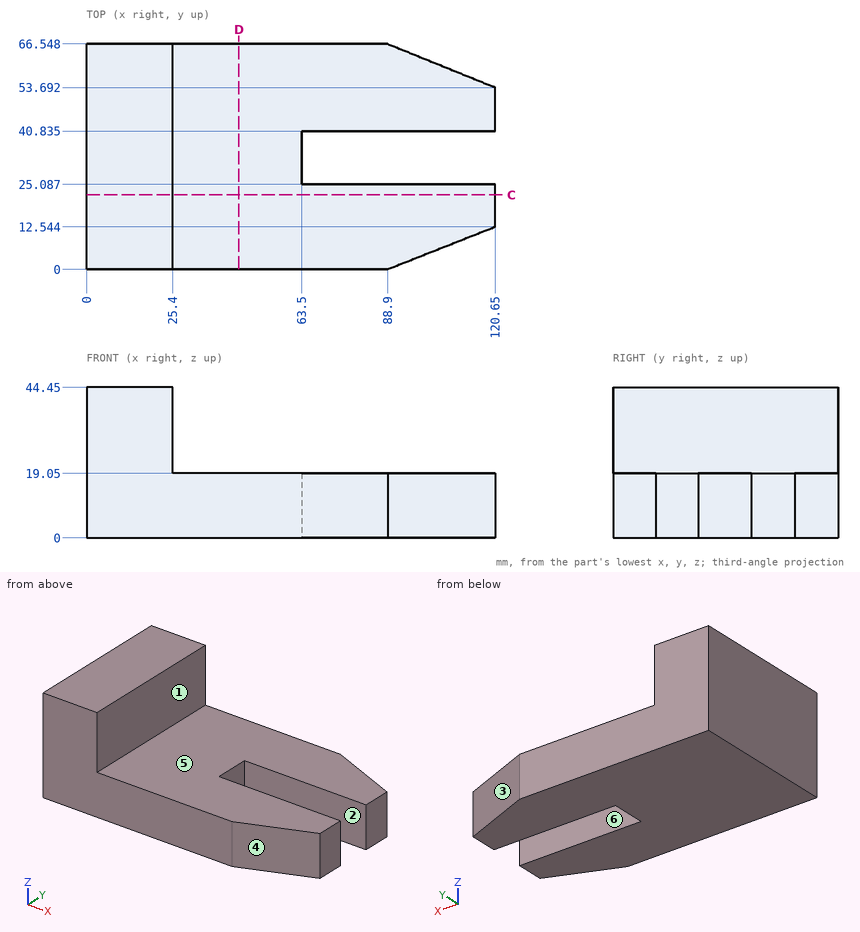
The drawing under review shows one solid part. Ordinate dimensions are in mm from its lowest x, y, z. A direction names the side the tool comes from. Coordinates: 2 decimals unless noted, no trailing zeros. Order: outer loops, then holes, each group sorted by start corner. A loop starts at its lowest first (then second) coordinate and runs counter-clockwise, first axis right, second up. Notation, with made-up numbers: (28.5, 6.5) -> (62.5, 6.5) arc R28 cw to (62.5, 26.5) -> close; hole circle Ø2 at (-5, -28). An arc over 180 degrees is marked (long way). Answer as CSV lines item,"result".
Q1. We need section D-D (x = 45). State the section outline as (y, z) points, plus the area to 3 significant figures.
Model answer:
outline,"(0, 0) -> (66.55, 0) -> (66.55, 19.05) -> (0, 19.05) -> close"
area,"1,270 mm2"
Q2. For the marked faces 1, 2 and 3, list the 3-axis set-ups (+Z, -Z, +X, -X, +Y, -Y) from which the entire face can be reached by the end or side of a thin tool; tool diameter is ignored.
Model answer:
face 1,"+Z, +X, +Y, -Y"
face 2,"+Z, -Z, +X"
face 3,"+Z, -Z, +X, +Y"
Q3. We need section C-C (y = 22). State the section outline as (x, z) points.
Model answer:
outline,"(0, 0) -> (120.65, 0) -> (120.65, 19.05) -> (25.4, 19.05) -> (25.4, 44.45) -> (0, 44.45) -> close"
Q4. Draft analysis for pull direction Y (two halves, no side actions). For the marked faces 4, 5 and 6, state which applies: released by +Y, released by -Y, zero draft, split by the parting line, or undercut.
Model answer:
face 4,"released by -Y"
face 5,"zero draft"
face 6,"undercut"
Q5. Clearance check with flat-ended pins moving along their axes: pin 1 Ø5.5 at (x, z) = (105, 13) entering from +Y; pin 2 Ø2 at (x, y) = (92, 10.5) entering from +Z; pin 3 Ø12 at (x, z) = (95, 4.5) entering from -Y. State where each tip first meets the part, or that it passes through.
Model answer:
pin 1,"stops at y = 61.14"
pin 2,"stops at z = 19.05"
pin 3,"stops at y = 0.04"
Q6. Wall thickness on line 1 along Y through (x, z) = (68, 12) (1 decimal); line 2 along X through (y, z) = (56, 40.5); line 3 along Y through (x, z) = (92.5, 18) (1 decimal): over which ranges is each line inside the solid? List them lowest first. Write a range as [from, to].
Model answer:
line 1,"y = [0, 25.1], [40.8, 66.5]"
line 2,"x = [0, 25.4]"
line 3,"y = [1.4, 25.1], [40.8, 65.1]"
